Can you work these out from the model? Positions are in its coordinate system, mm. Round coordinates to 2 decimals unless told otherwise and drop trailing zeros. Write each loop counter-clockwise with the first axis right and the second up, starting at its lowest first coordinate (ties: lowest second). Pieces come first, ordered by that corner, then holes. Notation, with made-up numbers: (23.25, 0) -> (75.25, 0) arc R15 cw to (75.25, 17) -> close; hole circle Ø9 at (-28, 49). An arc over 180 degrees is marked (long way). Write item = value, one per line. Start each with the question number.
1) If I drill on line 1 (Y direction, x = -15.5, z = -0.75); line 2 (Y direction, x = 0, z = -0.9); line 3 (X direction, y = -14.5, z = -0.2), over which ranges is the centre line in solid material (lowest first)?
2) Imagine slicing it at D-D, the plane x = 17. Please give me the cut outline in (y, z).
3) Imagine slicing it at C-C, the plane z = -0.7. State how many separate pieces and enclosed holes the cut face has, then the cut area to 3 significant figures.
4) Imagine slicing it at A-A, the plane y = 0. Please give me the cut outline in (x, z).
5) Imagine slicing it at B-B, the plane x = 10. Please give me the cut outline in (y, z), then the cut area to 3 significant figures.
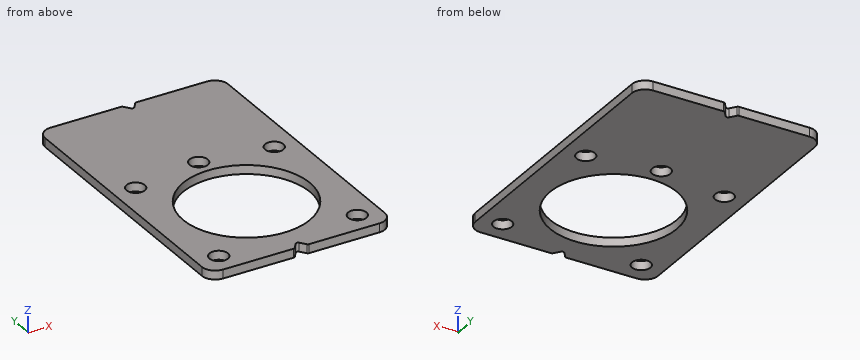
from build123d import *

# Parameters (mm, degrees)
SKETCH2_R               = 20.6375
SKETCH2_R_2             = 14.2875
BOSS_EXTRUDE1_DEPTH     = 1
CUT_EXTRUDE1_DEPTH      = 49.96874322
CUT_EXTRUDE1_DEPTH_BACK = 49.96874322
SKETCH3_R               = 2.07
FILLET1_R               = 3
FILLET3_R               = 0.5


with BuildPart() as part:
    # Sketch2 → Boss-Extrude1 (new, symmetric)
    # profile 1 of 4: a face of its own
    with BuildSketch(Plane.XY):
        Circle(SKETCH2_R)
        Circle(SKETCH2_R_2, mode=Mode.SUBTRACT)
    # profile 2 of 4: a face of its own
    with BuildSketch(Plane.XY):
        with BuildLine():
            Line((-20.6375, 44.3625), (-20.6375, 0))
            ThreePointArc((-20.6375, 0), (0, 20.6375), (20.6375, 0))
            Line((20.6375, 0), (20.6375, 44.3625))
            Line((20.6375, 44.3625), (-20.6375, 44.3625))
        make_face()
    # profile 3 of 4: a face of its own
    with BuildSketch(Plane.XY):
        with BuildLine():
            ThreePointArc((20.6375, 0), (14.592916166, -14.592916227), (-8.6e-08, -20.6375))
            Line((-8.6e-08, -20.6375), (20.6375, -20.6375))
            Line((20.6375, -20.6375), (20.6375, 0))
        make_face()
    # profile 4 of 4: a face of its own
    with BuildSketch(Plane.XY):
        with BuildLine():
            Line((-20.6375, 0), (-20.6375, -20.6375))
            Line((-20.6375, -20.6375), (-8.6e-08, -20.6375))
            ThreePointArc((-8.6e-08, -20.6375), (-14.592916227, -14.592916166), (-20.6375, 0))
        make_face()
    extrude(amount=BOSS_EXTRUDE1_DEPTH, both=True)

    # Sketch3 → Cut-Extrude1 (cut, two sides: drawn at the far end of the back side and taken through both)
    with BuildSketch(Plane.XY.offset(1).offset(-CUT_EXTRUDE1_DEPTH_BACK)):
        with Locations((0, 18)):
            Circle(SKETCH3_R)
        with Locations((-15.6375, -15.6375)):
            Circle(SKETCH3_R)
        with Locations((15.6375, -15.6375)):
            Circle(SKETCH3_R)
        with Locations((15.6375, 15.6375)):
            Circle(SKETCH3_R)
        with Locations((-15.6375, 15.6375)):
            Circle(SKETCH3_R)
        Polygon((0, 44.3625), (-1.5, 44.3625), (0, 42.3625), (1.5, 44.3625), align=None)
        Polygon((1.5, -20.6375), (0, -18.6375), (-1.5, -20.6375), (0, -20.6375), align=None)
    extrude(amount=CUT_EXTRUDE1_DEPTH + CUT_EXTRUDE1_DEPTH_BACK, mode=Mode.SUBTRACT)

    # Fillet1
    fillet1_edges = [part.edges().sort_by_distance(p)[0] for p in [
        (-20.6375, -20.6375, 0),
        (-20.6375, 44.3625, 0),
        (20.6375, 44.3625, 0),
        (20.6375, -20.6375, 0),
    ]]
    fillet(fillet1_edges, radius=FILLET1_R)

    # Fillet3
    fillet3_edges = [part.edges().sort_by_distance(p)[0] for p in [
        (1.5, -20.6375, 0),
        (-1.5, -20.6375, 0),
        (0, -18.6375, 0),
        (1.5, 44.3625, 0),
        (0, 42.3625, 0),
        (-1.5, 44.3625, 0),
    ]]
    fillet(fillet3_edges, radius=FILLET3_R)


solid = part.part
Reported:
q1.line_1 = -20.64 to -17.7, -13.57 to 13.57, 17.7 to 44.36
q1.line_2 = -18.97 to -14.29, 14.29 to 15.93, 20.07 to 42.7
q1.line_3 = -20.64 to -17.37, -13.91 to 13.91, 17.37 to 20.64
q2.outline = (-20.64, -1) -> (-17.2, -1) -> (-17.2, 1) -> (-20.64, 1) -> close; (-14.08, -1) -> (14.08, -1) -> (14.08, 1) -> (-14.08, 1) -> close; (17.2, -1) -> (44.36, -1) -> (44.36, 1) -> (17.2, 1) -> close
q3.separate_pieces = 1
q3.enclosed_holes = 6
q3.area = 1,960 mm²
q4.outline = (-20.64, -1) -> (-14.29, -1) -> (-14.29, 1) -> (-20.64, 1) -> close; (14.29, -1) -> (20.64, -1) -> (20.64, 1) -> (14.29, 1) -> close
q5.outline = (-20.64, -1) -> (-10.2, -1) -> (-10.2, 1) -> (-20.64, 1) -> close; (10.2, -1) -> (44.36, -1) -> (44.36, 1) -> (10.2, 1) -> close
q5.area = 89.2 mm²
